Check sheet for the modelled part. Datum: model origin and axes. Units: mm. Face numbers are marked on the shaded views. Round coordinates to 2 decimals unless told otherwise and drop trailing zeros. Loops run counter-clockwise (first coordinate to the right, second up) from the corner with the lowest first, then second, coordinate; pieces in that order, holes last. Notation, with made-up numbers: (46.25, -37) - (93.25, -37) arc R20 ccw to (93.25, -31) - close; hole circle Ø2 at (-35, 14.25). An arc over 180 degrees is marked (long way). Answer in a Markdown table with one row per item. Add a question column.
(1) Cross-section at D-D on x = 1.7. Enter the section's corners in (y, z), then the cut area to 3 significant figures.
(2) Cross-section at C-C on y = -0.25. Enter the section's corners in (x, z).
(3) Cross-section at B-B on z = 3.25. Enter the section's corners in (x, y).
(4) Thickness scan on line 1 along Y through (x, z) = (0, 1.75); line 2 along X through (y, z) = (2.25, 2.75); line 3 along X through (y, z) = (0, 3). Record the ranges inside material, lowest first.
(5) Mould release check, pull along Y, two halves, no side actions. Record for the marked faces 1, 2, 3 and 4: +Y half, -Y half, draft (parallel to the pull), parting line (faces both ways), or undercut.
(6) Cross-section at A-A on x = 0. Enter the section's corners in (y, z).
from build123d import *

# Parameters (mm, degrees)
F0_W     = 4.8
F0_H     = 7.8
F0_R     = 1.25
F1_DEPTH = 8
F2_R     = 1.75


with BuildPart() as f1:
    # F0 (on Top) → F1 (new body)
    with BuildSketch(Plane.XY):
        Rectangle(F0_W, F0_H)
        with Locations((0, -0.25)):
            Circle(F0_R, mode=Mode.SUBTRACT)
    extrude(amount=F1_DEPTH)

    # F2
    f2_edges = [f1.edges().sort_by_distance(p)[0] for p in [
        (-2.4, -3.9, 4),
        (2.4, -3.9, 4),
        (2.4, 3.9, 4),
        (-2.4, 3.9, 4),
    ]]
    fillet(f2_edges, radius=F2_R)


solid = f1.part
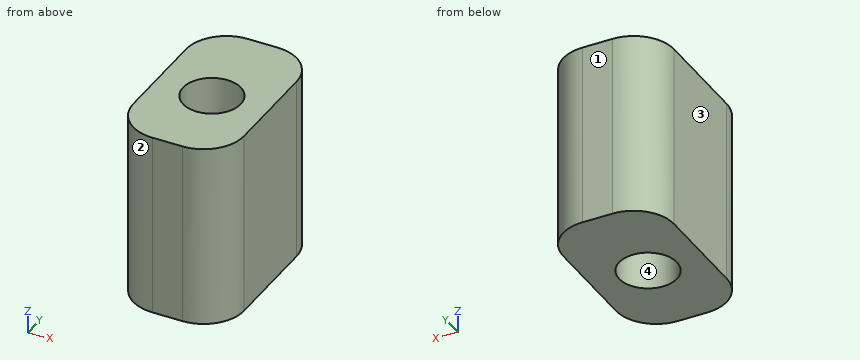
Answers:
| question | item | result |
|---|---|---|
| 1 | outline | (-3.55, 0) - (3.55, 0) - (3.55, 8) - (-3.55, 8) - close |
| 1 | area | 56.8 mm^2 |
| 2 | outline | (-2.4, 0) - (-1.25, 0) - (-1.25, 8) - (-2.4, 8) - close; (1.25, 0) - (2.4, 0) - (2.4, 8) - (1.25, 8) - close |
| 3 | outline | (-2.4, -2.15) arc R1.75 ccw to (-0.65, -3.9) - (0.65, -3.9) arc R1.75 ccw to (2.4, -2.15) - (2.4, 2.15) arc R1.75 ccw to (0.65, 3.9) - (-0.65, 3.9) arc R1.75 ccw to (-2.4, 2.15) - close; hole circle Ø2.5 at (0, -0.25) |
| 4 | line 1 | y = -3.9 to -1.5, 1 to 3.9 |
| 4 | line 2 | x = -2.4 to 2.4 |
| 4 | line 3 | x = -2.4 to -1.22, 1.22 to 2.4 |
| 5 | face 1 | +Y half |
| 5 | face 2 | -Y half |
| 5 | face 3 | draft |
| 5 | face 4 | undercut |
| 6 | outline | (-3.9, 0) - (-1.5, 0) - (-1.5, 8) - (-3.9, 8) - close; (1, 0) - (3.9, 0) - (3.9, 8) - (1, 8) - close |
